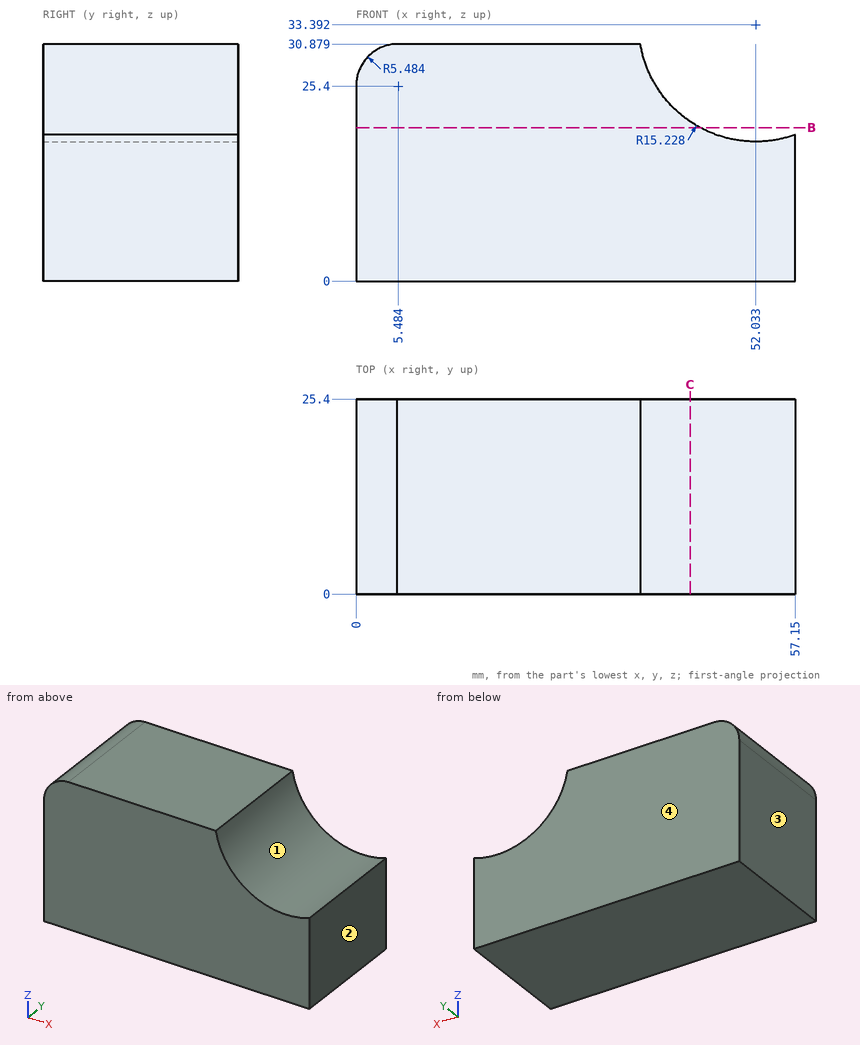
Geometry check sheet. Reference: drawing and pictorial views, mm from the part's lowest x, y, z. Give positions to 0.01 mm unless a question says otherwise; leave off trailing zeros. Order: outer loops, then holes, each group sorted by start corner. A loop starts at its lowest first (then second) coordinate and runs counter-clockwise, first axis right, second up.
1. Gauge pin test, flat ends, axial feed: pin 1 Ø3 at (y, z) = (4, 21) entering from +X (1 decimal); pin 2 Ø1 at (x, y) = (46, 8) entering from +Z; pin 3 Ø3 at (y, z) = (12, 23.5) entering from +X. Record the tip position at first contact, or that the pin passes through.
2. Release check for a two-part mould opening along X. For the marked faces 1, 2, 3 and 4 record: pulls with the +X half, pulls with the -X half, needs draft (parallel to the pull), parting line crosses it, or undercut.
3. Section check C-C, the plane x = 43.5. Enter the section's corners in (y, z).
4. Section check B-B, the plane z = 20. Enter the section's corners in (x, y) (1 decimal).
5. Thickness scan on L1, parallel to Z at x = 52, y = 12.5 (1 decimal); L2, parallel to Z at x = 3.5, y = 6.25; L3, parallel to X at y = 19.5, z = 21 (1 decimal). Record the ranges inside material, lowest first.
Values follow:
1. pin 1: stops at x = 45.8
1. pin 2: stops at z = 19.64
1. pin 3: stops at x = 41.93
2. face 1: undercut
2. face 2: pulls with the +X half
2. face 3: pulls with the -X half
2. face 4: needs draft
3. outline: (0, 0) - (25.4, 0) - (25.4, 20.78) - (0, 20.78) - close
4. outline: (0, 0) - (44.8, 0) - (44.8, 25.4) - (0, 25.4) - close
5. L1: z = 0 to 18.2
5. L2: z = 0 to 30.51
5. L3: x = 0 to 43.2
